from build123d import *

# Parameters (mm, degrees)
SKETCH1_R             = 30
SKETCH1_R_2           = 15
BOSS_EXTRUDE1_DEPTH   = 7.53
F_1_0MM_DOWEL_HOLE1_D = 4
CIRPATTERN1_COUNT     = 8


with BuildPart() as part:
    # Sketch1 → Boss-Extrude1 (new body)
    with BuildSketch(Plane.XY):
        Circle(SKETCH1_R)
        Circle(SKETCH1_R_2, mode=Mode.SUBTRACT)
    extrude(amount=BOSS_EXTRUDE1_DEPTH)

    # Ø1.0mm Dowel Hole1 (through all)
    with Locations(Plane.XY.offset(7.53)):
        with Locations((0, 26)):
            f_1_0mm_dowel_hole1 = Hole(F_1_0MM_DOWEL_HOLE1_D / 2)

    # CirPattern1: Ø1.0mm Dowel Hole1 ×8 about axis
    cirpattern1_axis = Axis((0, 0, 0), (0, 0, 1))
    for i in range(1, CIRPATTERN1_COUNT):
        add(f_1_0mm_dowel_hole1.rotate(cirpattern1_axis, i * 360 / CIRPATTERN1_COUNT), mode=Mode.SUBTRACT)


solid = part.part
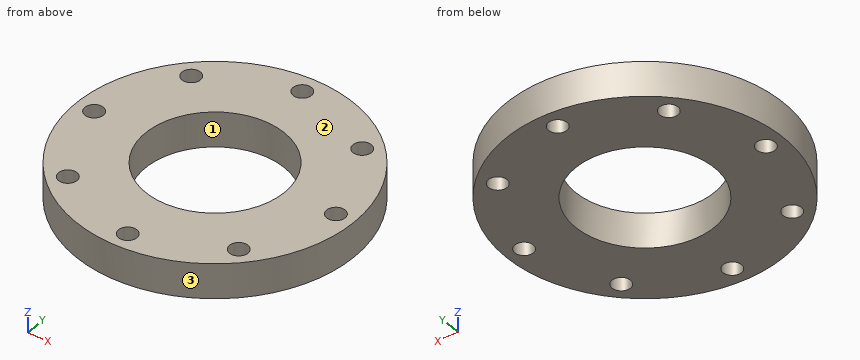
Could you check a few things on this model? Use its own coordinates, in mm. Face numbers are marked on the shaded views. Round coordinates to 2 decimals unless told otherwise and drop trailing zeros. Write each loop counter-clockwise with the first axis right and the second up, starting at its lowest first coordinate (ties: lowest second). Pieces come first, ordered by that corner, then holes. Notation, with made-up numbers: (36, 67.5) - (63, 67.5) arc R14 cw to (63, 87.5) - close; hole circle Ø1 at (-23, 30.25). An arc over 180 degrees is marked (long way). Put each result on its own line as item: value. Start each with the question number.
(1) I want a section at A-A, the plane x = 0. Please give me the cut outline in (y, z).
(2) Thinking about a two-plate mould opening in Y: for the marked faces 1, 2 and 3, which applies, released by +Y, released by -Y, zero draft, split by the parting line, or undercut?
(3) I want a section at C-C, the plane z = 1.75. Give the number of separate pieces and of enclosed holes in the cut face, plus the area to 3 significant figures.
(4) I need wall thicknesses on probe 1 along Y at (x, z) = (0, 5.25); probe 2 along Y at (x, z) = (18.5, 4.5); probe 3 along X at (y, z) = (-18, 3.5). Which ranges of each line are inside material? Lowest first, please.
(5) Will these pins go through, and if not, where does the flat tip stop? pin 1 (2 mm diameter, centred on y = 8, z = 3, fed in from +X); pin 2 (4 mm diameter, centred on y = 2.5, z = 3.5, fed in from +X).
(6) I want a section at D-D, the plane y = 10. Please give me the cut outline in (x, z).
Here are the results:
1. outline: (-30, 0) - (-28, 0) - (-28, 7.53) - (-30, 7.53) - close; (-24, 0) - (-15, 0) - (-15, 7.53) - (-24, 7.53) - close; (15, 0) - (24, 0) - (24, 7.53) - (15, 7.53) - close; (28, 0) - (30, 0) - (30, 7.53) - (28, 7.53) - close
2. face 1: undercut
2. face 2: zero draft
2. face 3: split by the parting line
3. separate pieces: 1
3. enclosed holes: 9
3. area: 2,020 mm^2
4. probe 1: y = -30 to -28, -24 to -15, 15 to 24, 28 to 30
4. probe 2: y = -23.62 to -20.38, -16.39 to 16.39, 20.38 to 23.62
4. probe 3: x = -24 to -20.35, -16.42 to 16.42, 20.35 to 24
5. pin 1: stops at x = 29.17
5. pin 2: stops at x = 30
6. outline: (-28.28, 0) - (-11.18, 0) - (-11.18, 7.53) - (-28.28, 7.53) - close; (11.18, 0) - (28.28, 0) - (28.28, 7.53) - (11.18, 7.53) - close
